Could you check a few things on this model? Use its own coordinates, in mm. A direction names the side the tool comes from. Coordinates: 2 decimals unless noted, no trailing zeros. Loops run counter-clockwise (first coordinate to the right, second up) from the corner with the lowest first, then second, coordinate; pieces in that order, holes last. Notation, with made-up numbers: M 80,57.5 L 106,57.5 A10 ccw 106,75.5 Z; hole C -3.75,-32 d8. An arc over 180 degrees is marked long. Write each question's results on one line, items separated by ' | '.
Autodesk Inventor part; units mm, degrees
ref_plane "YZ Plane" through (0, 0, 0) normal (1, 0, 0) x (0, 1, 0)
ref_plane "XZ Plane" through (0, 0, 0) normal (0, 1, 0) x (-1, 0, 0)
ref_plane "XY Plane" through (0, 0, 0) normal (0, 0, 1) x (1, 0, 0)
sketch "Boceto1" plane through (0, 0, 0) normal (0, 1, 0) x (-1, 0, 0)
  line L0 (12.565, 24) -> (-13.135, 24)
  line L1 (-13.135, 24) -> (-13.135, -24)
  line L2 (-13.135, -24) -> (12.565, -24)
  line L3 (12.565, -24) -> (12.565, 24)
  point P0 (0, 0)
  point P1 (-0.285, -24)
  dimension "d0" = 48
  dimension "d1" = 25.7
  dimension "d2" = 12.565
  dimension "d3" = 24
extrude "Extrusión1" add sketch "Boceto1" along normal blind 5
fillet "Empalme1" radius 4 3 edges at (13.135, 2.5, 24) (13.135, 2.5, -24) (-12.565, 2.5, 24)
fillet "Empalme2" radius 4 1 edges at (-12.565, 2.5, -24)
sketch "Boceto2" plane through (0, 5, 0) normal (0, 1, 0) x (1, 0, 0)
  circle A0 centre (-9.865, -21.3) radius 1.5
  line L0 (-8.565, -24) -> (9.135, -24)
  line L1 (-12.565, 20) -> (-12.565, -20)
  line L2 (-31.929, 0) -> (35.0281, 0)
  circle A1 centre (-9.865, 21.3) radius 1.5
  line L3 (0.285, 24.6166) -> (0.285, -27.3805)
  circle A2 centre (10.435, -21.3) radius 1.5
  circle A3 centre (10.435, 21.3) radius 1.5
  line L4 (13.135, -20) -> (13.135, 20)
  line L5 (9.135, 24) -> (-8.565, 24)
  point P0 (0, 0)
  dimension "d8" = 3
  dimension "d9" = 2.7
  dimension "d10" = 2.7
  dimension "d21" = 2.7
  dimension "d22" = 2.7
extrude "Extrusión2" cut sketch "Boceto2" against normal blind 10
sketch "Boceto3" plane through (0, 0, 0) normal (0, -1, 0) x (1, 0, 0)
  line L0 (-11.565, 18.75) -> (-9.065, 18.75)
  line L1 (-9.065, 18.75) -> (-9.065, -18.75)
  line L2 (-9.065, -18.75) -> (-11.565, -18.75)
  line L3 (-11.565, -18.75) -> (-11.565, 18.75)
  line L4 (0.285, 27.3547) -> (0.285, -28.7593)
  line L5 (-12.565, -20) -> (-12.565, 20)
  line L6 (-8.565, 24) -> (9.135, 24)
  line L7 (9.135, -24) -> (-8.565, -24)
  line L8 (12.135, 18.75) -> (9.635, 18.75)
  line L9 (9.635, 18.75) -> (9.635, -18.75)
  line L10 (9.635, -18.75) -> (12.135, -18.75)
  line L11 (12.135, -18.75) -> (12.135, 18.75)
  line L12 (13.135, 20) -> (13.135, -20)
  point P0 (0, 0)
  point P1 (-10.315, 18.75)
  point P2 (-10.315, -18.75)
  point P3 (10.885, 18.75)
  point P4 (10.885, -18.75)
  dimension "d13" = 37.5
  dimension "d14" = 2.5
  dimension "d15" = 1
  dimension "d16" = 5.25
  dimension "d17" = 5.25
  dimension "d18" = 1
extrude "Extrusión3" add sketch "Boceto3" along normal blind 8
equation "\"Radio_pliegue\" = Grosor"
equation "\"Anchura_desahogo_plegado\" = Grosor"
equation "\"Profundidad_desahogo_plegado\" = 0.5 * Grosor"
equation "\"Tamaño_destalonado\" = 4 * Grosor"
equation "\"Remanente_mínimo\" = 2 * Grosor"
equation "\"Radiodetransición\" = Radio_pliegue"
equation "\"Tamaño_de_radio_de_Jacobi\" = Radio_pliegue"
equation "\"TamañoSeparación\" = Grosor"
properties part number "ESP_8266"
(1) Imagine slicing it at D-D, the plane z = -21.3. List the corners of the cut face in (x, y) for me (3 decimals).
Reported:
outline: M -12.348,0 L -11.365,0 L -11.365,5 L -12.348,5 Z; M -8.365,0 L 8.935,0 L 8.935,5 L -8.365,5 Z; M 11.935,0 L 12.918,0 L 12.918,5 L 11.935,5 Z
(2) If we mould it in two halves opening along X, with no side actions, what happens to faces 1 (the flat face through (0, 5, 0)), 2 (the cylindrical face through (-10.971, 2.535, 20.286)), 3 (the cylindrical face through (11.13, 2.54, -19.97)), 4 (the flat face through (13.135, 2, 0))? For each: released by +X, released by -X, zero draft, split by the parting line, or undercut.
Reported:
face 1: zero draft | face 2: undercut | face 3: undercut | face 4: released by +X
(3) Which directions (+Z, -Z, +X, -X, +Y, -Y) give clear straight access to the entire face, cutting with the end or side of a thin tool? Please do faces 5 (the flat face through (11, -4, -18.75)), 6 (the flat face through (0, 2, -24)), 7 (the flat face through (9.635, -4, 0)), 8 (the flat face through (12.135, -4, 0)), 9 (the flat face through (-10, -4, 18.75)).
Reported:
face 5: -Z, +X, -X, -Y | face 6: -Z, +X, -X, +Y, -Y | face 7: +Z, -Z, -Y | face 8: +Z, -Z, +X, -Y | face 9: +Z, +X, -X, -Y
(4) Please list where these lines run through material, in increasing order: probe 1 along X at (y, z) = (-2, -13.5) (3 decimals); probe 2 along X at (y, z) = (2.15, 21.3) (3 decimals); probe 3 along Y at (x, z) = (7, 9.5). Write a range as from..to.
Reported:
probe 1: x = -11.565..-9.065, 9.635..12.135 | probe 2: x = -12.348..-11.365, -8.365..8.935, 11.935..12.918 | probe 3: y = 0..5
(5) Imagine slicing it at A-A, the plane y = 0.75. List the corners of the cut face in (x, z) for me (3 decimals), and give its area (3 significant figures).
Reported:
outline: M -12.565,-20 A4 ccw -8.565,-24 L 9.135,-24 A4 ccw 13.135,-20 L 13.135,20 A4 ccw 9.135,24 L -8.565,24 A4 ccw -12.565,20 Z; hole C -9.865,-21.3 d3; hole C -9.865,21.3 d3; hole C 10.435,-21.3 d3; hole C 10.435,21.3 d3 | area: 1,190 mm2
(6) Imagine slicing it at B-B, the plane z = 17. List the corners of the cut face in (x, y) for me (3 decimals), and give its area (4 significant figures).
Reported:
outline: M -12.565,0 L -11.565,0 L -11.565,-8 L -9.065,-8 L -9.065,0 L 9.635,0 L 9.635,-8 L 12.135,-8 L 12.135,0 L 13.135,0 L 13.135,5 L -12.565,5 Z | area: 168.5 mm2
(7) Imagine slicing it at C-C, the plane y = -3.5. List the corners of the cut face in (x, z) for me (3 decimals), and give its area (4 significant figures).
Reported:
outline: M -11.565,-18.75 L -9.065,-18.75 L -9.065,18.75 L -11.565,18.75 Z; M 9.635,-18.75 L 12.135,-18.75 L 12.135,18.75 L 9.635,18.75 Z | area: 187.5 mm2
(8) Will these pins go through, and if not, where does the flat tip stop? P1, Ø7.5, axis at x = 5, z = 6.5, coming from the -Y side; P2, Ø4, axis at y = -6.5, z = -17.5, coming from the +X side (3 decimals); P3, Ø4, axis at y = -5.5, z = 1, coming from the -X side (3 decimals).
Reported:
P1: stops at y = 0 | P2: stops at x = 12.135 | P3: stops at x = -11.565
